Part model, mm, in its own coordinate system. Face numbers are marked on the shaded views. A direction names the side the tool comes from. Round coordinates to 2 decimals unless told otherwise and drop trailing zeros. Loops run counter-clockwise (first coordinate to the right, second up) from the corner with the lowest first, then second, coordinate; pieces in that order, holes last.
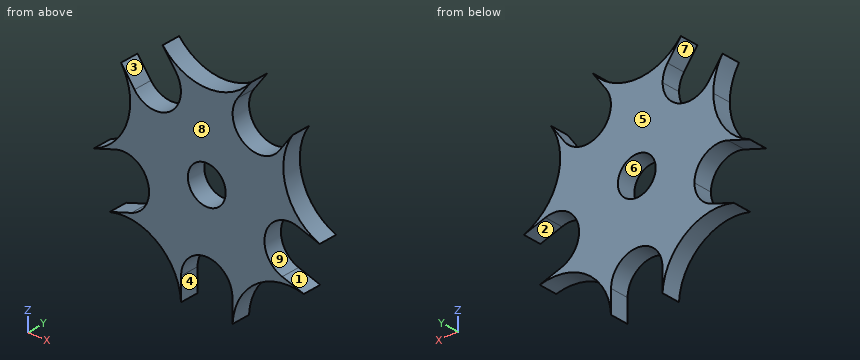
from build123d import *

# Parameters (mm, degrees)
F0_R     = 6.35
F1_DEPTH = 6.35


with BuildPart() as f1:
    # F0 (on Front) → F1 (new body)
    with BuildSketch(Plane.XZ):
        with BuildLine():
            ThreePointArc((8.63127, -37.109449), (8.644315, -37.106412), (8.657358, -37.103371))
            ThreePointArc((8.657358, -37.103371), (16.483961, -22.688226), (32.612132, -19.699209))
            ThreePointArc((32.612132, -19.699209), (32.619055, -19.687744), (32.625974, -19.676276))
            Line((32.625974, -19.676276), (25.359218, -17.315164))
            ThreePointArc((25.359218, -17.315164), (19.817602, -6.439129), (30.693637, -0.897512))
            Line((30.693637, -0.897512), (37.960392, -3.258624))
            ThreePointArc((37.960392, -3.258624), (37.961535, -3.24528), (37.962674, -3.231935))
            ThreePointArc((37.962674, -3.231935), (26.67161, 8.666131), (28.812764, 24.92859))
            ThreePointArc((28.812764, 24.92859), (28.803999, 24.938717), (28.795231, 24.948841))
            Line((28.795231, 24.948841), (24.304129, 18.76737))
            ThreePointArc((24.304129, 18.76737), (12.247951, 16.857859), (10.33844, 28.914037))
            Line((10.33844, 28.914037), (14.829542, 35.095508))
            ThreePointArc((14.829542, 35.095508), (14.817204, 35.100719), (14.804864, 35.105925))
            ThreePointArc((14.804864, 35.105925), (0, 28.04419), (-14.804864, 35.105925))
            ThreePointArc((-14.804864, 35.105925), (-14.817204, 35.100719), (-14.829542, 35.095508))
            Line((-14.829542, 35.095508), (-10.33844, 28.914037))
            ThreePointArc((-10.33844, 28.914037), (-9.112459, 26.507912), (-8.690014, 23.840703))
            ThreePointArc((-8.690014, 23.840703), (-14.654076, 15.631877), (-24.304129, 18.76737))
            Line((-24.304129, 18.76737), (-28.795231, 24.948841))
            ThreePointArc((-28.795231, 24.948841), (-28.803999, 24.938717), (-28.812764, 24.92859))
            ThreePointArc((-28.812764, 24.92859), (-26.523773, 19.963575), (-25.739236, 14.552905))
            ThreePointArc((-25.739236, 14.552905), (-29.089738, 3.762713), (-37.962674, -3.231935))
            ThreePointArc((-37.962674, -3.231935), (-37.961535, -3.24528), (-37.960392, -3.258624))
            Line((-37.960392, -3.258624), (-30.693637, -0.897512))
            ThreePointArc((-30.693637, -0.897512), (-22.953094, -2.123494), (-19.395157, -9.106338))
            ThreePointArc((-19.395157, -9.106338), (-21.043583, -14.179672), (-25.359218, -17.315164))
            Line((-25.359218, -17.315164), (-32.625974, -19.676276))
            ThreePointArc((-32.625974, -19.676276), (-32.619055, -19.687744), (-32.612132, -19.699209))
            ThreePointArc((-32.612132, -19.699209), (-16.483961, -22.688226), (-8.657358, -37.103371))
            ThreePointArc((-8.657358, -37.103371), (-8.644315, -37.106412), (-8.63127, -37.109449))
            Line((-8.63127, -37.109449), (-8.63127, -29.46873))
            ThreePointArc((-8.63127, -29.46873), (0, -20.837459), (8.63127, -29.46873))
            Line((8.63127, -29.46873), (8.63127, -37.109449))
        make_face()
        Circle(F0_R, mode=Mode.SUBTRACT)
    extrude(amount=F1_DEPTH)


solid = f1.part
1) Mould opens along X. For the marked faces 6, 7, 8 and 9 say: released by +X, released by -X, zero draft, split by the parting line, or undercut.
Values:
face 6: undercut
face 7: released by -X
face 8: zero draft
face 9: undercut
2) Wall check: line 1 along Z through (x, y) = (0, -3); line 2 along Z through (x, y) = (-2.5, -4.5); line 3 along X through (y, z) = (-5, 23.5). Give the ranges that are in metal, low to high.
Values:
line 1: z = -20.84 to -6.35, 6.35 to 28.04
line 2: z = -21.21 to -5.84, 5.84 to 28.21
line 3: x = -27.97 to -27.74, -8.7 to 8.7, 27.74 to 27.97
3) Slice it at C-C, the plane x = -13. Give the cut face in (y, z), then the cut area to 3 significant figures.
Values:
outline: (-6.35, -25.96) - (0, -25.96) - (0, 16.37) - (-6.35, 16.37) - close; (-6.35, 32.58) - (0, 32.58) - (0, 33.17) - (-6.35, 33.17) - close
area: 273 mm2
4) Tool access for the marked faces 1, 2, 3, 4 and 5: list every direction of +Z, -Z, +X, -X, +Y, -Y with a clear straight run to the whole face (end or side of a thin tool).
Values:
face 1: +X, +Y, -Y
face 2: +Y, -Y
face 3: +Z, +Y, -Y
face 4: -Z, +Y, -Y
face 5: +Z, -Z, +X, -X, +Y
5) Slice it at A-A, the plane x = 0. Give the cut face in (y, z), then the cut area to 3 significant figures.
Values:
outline: (-6.35, -20.84) - (0, -20.84) - (0, -6.35) - (-6.35, -6.35) - close; (-6.35, 6.35) - (0, 6.35) - (0, 28.04) - (-6.35, 28.04) - close
area: 230 mm2
6) Drop a flat-ended pin along its axis: pin 1 Ø1.9 at (y, z) = (-4, -32.5) entering from +X. Give the stop position or say it passes through.
Values:
pin 1: stops at x = 9.79
